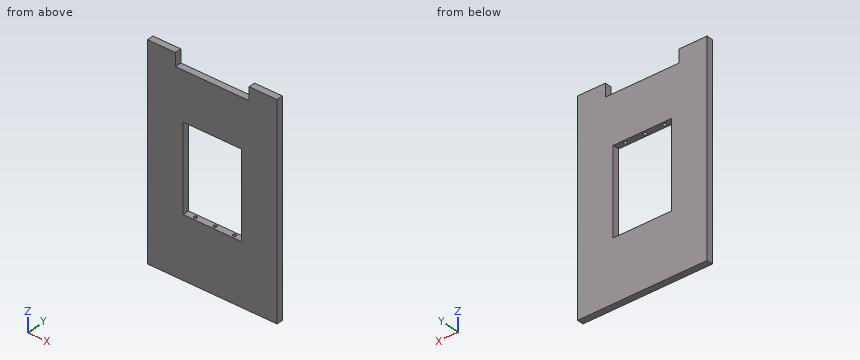
from build123d import *

# Parameters (mm, degrees)
SKETCH1_W                 = 100
SKETCH1_H                 = 160
BOSS_EXTRUDE1_DEPTH       = 5
SKETCH2_W                 = 45
SKETCH2_H                 = 66
CUT_EXTRUDE1_DEPTH        = 95.472218138
F_2_5MM_DOWEL_HOLE1_D     = 2.5
F_2_5MM_DOWEL_HOLE1_DEPTH = 10
F_2_5MM_DOWEL_HOLE1_TIP   = 0.751075774
F_2_5MM_DOWEL_HOLE2_D     = 2.5
F_2_5MM_DOWEL_HOLE2_DEPTH = 10
F_2_5MM_DOWEL_HOLE2_TIP   = 0.751075774
SKETCH8_W                 = 57
SKETCH8_H                 = 20
CUT_EXTRUDE2_DEPTH        = 95.472218138


with BuildPart() as part:
    # Sketch1 → Boss-Extrude1 (new body)
    with BuildSketch(Plane(origin=(0, 0, 0), x_dir=(1, 0, 0), z_dir=(0, 1, 0))):
        Rectangle(SKETCH1_W, SKETCH1_H)
    extrude(amount=BOSS_EXTRUDE1_DEPTH)

    # Sketch2 → Cut-Extrude1 (cut, through all)
    with BuildSketch(Plane(origin=(0, 5, 0), x_dir=(1, 0, 0), z_dir=(0, 1, 0))):
        Rectangle(SKETCH2_W, SKETCH2_H)
    extrude(amount=-CUT_EXTRUDE1_DEPTH, mode=Mode.SUBTRACT)

    # Ø2.5mm Dowel Hole1
    with Locations(Plane.XY.offset(-33)):
        with Locations((0, 2.5), (15, 2.5), (-15, 2.5)):
            Hole(F_2_5MM_DOWEL_HOLE1_D / 2, depth=F_2_5MM_DOWEL_HOLE1_DEPTH)
            with Locations((0, 0, -(F_2_5MM_DOWEL_HOLE1_DEPTH + F_2_5MM_DOWEL_HOLE1_TIP / 2))):  # 118° drill point
                Cone(0, F_2_5MM_DOWEL_HOLE1_D / 2, F_2_5MM_DOWEL_HOLE1_TIP, mode=Mode.SUBTRACT)

    # Ø2.5mm Dowel Hole2
    with Locations(Plane(origin=(0, 0, 33), x_dir=(-1, 0, 0), z_dir=(0, 0, -1))):
        with Locations((0, 2.5), (15, 2.5), (-15, 2.5)):
            Hole(F_2_5MM_DOWEL_HOLE2_D / 2, depth=F_2_5MM_DOWEL_HOLE2_DEPTH)
            with Locations((0, 0, -(F_2_5MM_DOWEL_HOLE2_DEPTH + F_2_5MM_DOWEL_HOLE2_TIP / 2))):  # 118° drill point
                Cone(0, F_2_5MM_DOWEL_HOLE2_D / 2, F_2_5MM_DOWEL_HOLE2_TIP, mode=Mode.SUBTRACT)

    # Sketch8 → Cut-Extrude2 (cut, through all)
    with BuildSketch(Plane(origin=(0, 5, 0), x_dir=(1, 0, 0), z_dir=(0, 1, 0))):
        with Locations((0, -80)):
            Rectangle(SKETCH8_W, SKETCH8_H)
    extrude(amount=-CUT_EXTRUDE2_DEPTH, mode=Mode.SUBTRACT)


solid = part.part
Source: CAD feature listing. Evaluate the final solid. Frame: model axes, mm. Give positions to 0.01 mm unless a question says otherwise; leave off trailing zeros. Write each loop counter-clockwise with the first axis right and the second up, starting at its lowest first coordinate (ties: lowest second). Pieces come first, ordered by that corner, then holes. Notation, with made-up numbers: M 1.25,-0.5 L 33.25,-0.5 A19 cw 33.25,34.5 Z; hole C 57.25,-39.5 d11. An arc over 180 degrees is marked long. Return JSON: item names as keys, results as strings. Group by question number.
1) Material intervals for line 1 along X through (y, z) = (2.5, 40.25); line 2 along Y through (x, z) = (15, -35); line 3 along Z through (x, y) = (11.5, 3.75), sorted ascending. Write a range as [from, to].
2) Cut plane A-A, the plane z = 10. Output: boundary loops of the cut face in (x, y), plus the area to 3 significant figures.
3) Cut plane B-B, the plane x = 20. Output: boundary loops of the cut face in (y, z).
4) Pin query (flat end, axial travel): P1, Ø3, axis at x = 15, y = 2.5, coming from the +Z side. Return the tip coordinate at first contact, or that it passes through.
5) Cut plane C-C, the plane x = -24.5. Output: boundary loops of the cut face in (y, z).
Recorded:
{
 "1": {"line 1": "x = [-50, -16.25], [-13.75, -1.25], [1.25, 13.75], [16.25, 50]", "line 2": "y = [0, 1.25], [3.75, 5]", "line 3": "z = [-80, -33], [33, 70]"},
 "2": {"outline": "M -50,0 L -22.5,0 L -22.5,5 L -50,5 Z; M 22.5,0 L 50,0 L 50,5 L 22.5,5 Z", "area": "275 mm²"},
 "3": {"outline": "M 0,-80 L 5,-80 L 5,-33 L 0,-33 Z; M 0,33 L 5,33 L 5,70 L 0,70 Z"},
 "4": {"P1": "stops at z = 70"},
 "5": {"outline": "M 0,-80 L 5,-80 L 5,70 L 0,70 Z"}
}
